from build123d import *

# Parameters (mm, degrees)
CROQUIS1_R              = 2.005138112
SALIENTE_EXTRUIR1_DEPTH = 4
CROQUIS2_W              = 30
CROQUIS2_H              = 5
SALIENTE_EXTRUIR2_DEPTH = 30
CROQUIS3_R              = 1.75
CROQUIS3_R_2            = 4
CORTAR_EXTRUIR1_DEPTH   = 52.778373864
REDONDEO1_R             = 10
REDONDEO2_R             = 5
REDONDEO4_R             = 2
CROQUIS4_R              = 3.4
CORTAR_EXTRUIR2_DEPTH   = 2.25
NERVIO12_REACH          = 56.369
CROQUIS7_WALL_W         = 121.91855764
CROQUIS7_WALL_H         = 5
NERVIO13_REACH          = 56.369
CROQUIS8_WALL_W         = 121.91855764
CROQUIS8_WALL_H         = 5
REDONDEO6_R             = 3
REDONDEO7_R             = 2
REDONDEO8_R             = 1


with BuildPart() as part:
    # Croquis1 → Saliente-Extruir1 (new body)
    with BuildSketch(Plane.XY):
        Polygon((0, 21.15), (0, 30), (30, 30), (30, 21.15), (30, 14.85), (30, 0), (0, 0), (0, 14.85), align=None)
        with Locations((9, 18)):
            Circle(CROQUIS1_R, mode=Mode.SUBTRACT)
        with Locations((21, 18)):
            Circle(CROQUIS1_R, mode=Mode.SUBTRACT)
        with Locations((21, 6)):
            Circle(CROQUIS1_R, mode=Mode.SUBTRACT)
        with Locations((9, 6)):
            Circle(CROQUIS1_R, mode=Mode.SUBTRACT)
    extrude(amount=SALIENTE_EXTRUIR1_DEPTH)

    # Croquis2 → Saliente-Extruir2 (add)
    with BuildSketch(Plane.XY.offset(4)):
        with Locations((15, 27.5)):
            Rectangle(CROQUIS2_W, CROQUIS2_H)
    extrude(amount=SALIENTE_EXTRUIR2_DEPTH)

    # Croquis3 → Cortar-Extruir1 (cut, through all)
    with BuildSketch(Plane.XZ.offset(-25)):
        with Locations(Location((15, 27.25, 0), (0, 0, 270))):
            Circle(CROQUIS3_R)
        with Locations(Location((15, 10.75, 0), (0, 0, 270))):
            Circle(CROQUIS3_R)
        with Locations(Location((15, 19, 0), (0, 0, 270))):
            Circle(CROQUIS3_R_2)
    extrude(amount=-CORTAR_EXTRUIR1_DEPTH, mode=Mode.SUBTRACT)

    # Redondeo1
    redondeo1_edges = [part.edges().sort_by_distance(p)[0] for p in [
        (0, 27.5, 34),
        (30, 27.5, 34),
    ]]
    fillet(redondeo1_edges, radius=REDONDEO1_R)

    # Redondeo2
    redondeo2_edges = [part.edges().sort_by_distance(p)[0] for p in [
        (30, 0, 2),
        (0, 0, 2),
    ]]
    fillet(redondeo2_edges, radius=REDONDEO2_R)

    # Redondeo4
    redondeo4_edges = [part.edges().sort_by_distance(p)[0] for p in [
        (15, 30, 0),
    ]]
    fillet(redondeo4_edges, radius=REDONDEO4_R)

    # Croquis4 → Cortar-Extruir2 (cut)
    with BuildSketch(Plane(origin=(0, 30, 0), x_dir=(1, 0, 0), z_dir=(0, 1, 0))):
        with Locations(Location((15, -10.75, 0), (0, 0, 270))):
            Circle(CROQUIS4_R)
        with Locations(Location((15, -27.25, 0), (0, 0, 270))):
            Circle(CROQUIS4_R)
    extrude(amount=-CORTAR_EXTRUIR2_DEPTH, mode=Mode.SUBTRACT)

    # Croquis7 wall → Nervio12 (add, up to next)
    with BuildSketch(Plane(origin=(30, 20, 6.5), x_dir=(0, -0.894427191, -0.4472135955), z_dir=(0, 0.4472135955, -0.894427191)), mode=Mode.PRIVATE) as nervio12_sk1:
        with Locations((0, 2.5)):
            Rectangle(CROQUIS7_WALL_W, CROQUIS7_WALL_H)
    nervio12_tool1 = extrude(nervio12_sk1.sketch, amount=NERVIO12_REACH, mode=Mode.PRIVATE) - part.part
    add(nervio12_tool1.solids().sort_by_distance((30, 20, 6.5))[0])

    # Croquis8 wall → Nervio13 (add, up to next)
    with BuildSketch(Plane(origin=(0, 20, 6.5), x_dir=(0, 0.894427191, 0.4472135955), z_dir=(0, 0.4472135955, -0.894427191)), mode=Mode.PRIVATE) as nervio13_sk1:
        with Locations((0, 2.5)):
            Rectangle(CROQUIS8_WALL_W, CROQUIS8_WALL_H)
    nervio13_tool1 = extrude(nervio13_sk1.sketch, amount=NERVIO13_REACH, mode=Mode.PRIVATE) - part.part
    add(nervio13_tool1.solids().sort_by_distance((0, 20, 6.5))[0])

    # Redondeo6
    redondeo6_edges = [part.edges().sort_by_distance(p)[0] for p in [
        (27.5, 25, 9),
        (27.5, 15, 4),
        (2.5, 25, 9),
        (2.5, 15, 4),
    ]]
    fillet(redondeo6_edges, radius=REDONDEO6_R)

    # Redondeo7
    redondeo7_edges = [part.edges().sort_by_distance(p)[0] for p in [
        (15, 25, 4),
    ]]
    fillet(redondeo7_edges, radius=REDONDEO7_R)

    # Redondeo8
    redondeo8_edges = [part.edges().sort_by_distance(p)[0] for p in [
        (5, 25, 8.427050983),
        (5, 24.414213562, 4.585786438),
        (5, 18.645898034, 4),
        (25, 25, 8.427050983),
        (25, 24.414213562, 4.585786438),
        (25, 18.645898034, 4),
    ]]
    fillet(redondeo8_edges, radius=REDONDEO8_R)


solid = part.part
Check sheet for the modelled part. Datum: model origin and axes. Units: mm. A direction names the side the tool comes from. Round coordinates to 2 decimals unless told otherwise and drop trailing zeros. Order: outer loops, then holes, each group sorted by start corner. A loop starts at its lowest first (then second) coordinate and runs counter-clockwise, first axis right, second up.
(1) Cross-section at B-B, the plane y = 18. Enter the section's corners in (x, z), and give its area (3 significant figures).
(2) Cross-section at D-D, the plane y = 27.25. Enter the section's corners in (x, z).
(3) Cross-section at A-A, the plane z = 19. Enter the section's corners in (x, y).
(4) Go/stop test with flat-tipped pins: P1, Ø9, axis at x = 15, z = 10.75, coming from the -Y side; P2, Ø1.5, axis at x = 23.5, y = 15, coming from the +Z side; P3, Ø4, axis at x = 15, z = 27.25, coming from the +Y side; P4, Ø2.5, axis at x = 9, y = 18, coming from the +Z side. Record where each tip stops, or that it passes through.
(5) Scan lines: probe 1 along Y at (x, z) = (21, 2.85); probe 2 along X at (y, z) = (27, 10.75); probe 3 along Y at (x, z) = (9, 1). Record each from-to range of solid material in increasing order.
(6) Draft check along X on faces 1 (the flat face through (15, 0, 2)), 2 (the cylindrical face through (5.301, 19.553, 4.285)), 3 (the flat face through (16, 27.75, 9)), 4 (the cylindrical face through (28, 1, 2)). Enter one of: pulls with the +X half, pulls with the -X half, needs draft (parallel to the pull), parting line crosses it, or undercut.
(7) Cross-section at C-C, the plane x = 9. Enter the section's corners in (y, z), and give its area (3 significant figures).
(8) Access from +Z, -Z, +X, -X, +Y, -Y to the whole of each face (thin tool, end or side, straight path). Record for faces 5 (the cylindrical face through (11.68, 28.89, 10.01)), 6 (the flat face through (15, 9, 4)), 7 (the cylindrical face through (7.522, 19.355, 1.972)).
Check sheet entries:
1. outline: (0, 0) - (6.99, 0) - (6.99, 4) - (6, 4) arc R1 cw to (5, 5) - (5, 5.5) - (0, 5.5) - close; (11.01, 0) - (18.99, 0) - (18.99, 4) - (11.01, 4) - close; (23.01, 0) - (30, 0) - (30, 5.5) - (25, 5.5) - (25, 5) arc R1 cw to (24, 4) - (23.01, 4) - close
1. area: 103 mm2
2. outline: (0, 0) - (30, 0) - (30, 24) arc R10 ccw to (20, 34) - (10, 34) arc R10 ccw to (0, 24) - close; hole circle Ø8 at (15, 19); hole circle Ø3.5 at (15, 10.75); hole circle Ø3.5 at (15, 27.25)
3. outline: (0, 25) - (11, 25) - (11, 30) - (0, 30) - close; (19, 25) - (30, 25) - (30, 30) - (19, 30) - close
4. P1: stops at y = 25
4. P2: stops at z = 4.03
4. P3: stops at y = 27.75
4. P4: passes through
5. probe 1: y = 0 to 3.99, 8.01 to 15.99, 20.01 to 30
5. probe 2: x = 0 to 13.25, 16.75 to 30
5. probe 3: y = 0 to 3.99, 8.01 to 15.99, 20.01 to 29.73
6. face 1: needs draft
6. face 2: undercut
6. face 3: undercut
6. face 4: pulls with the +X half
7. outline: (0, 0) - (3.99, 0) - (3.99, 4) - (0, 4) - close; (8.01, 0) - (15.99, 0) - (15.99, 4) - (8.01, 4) - close; (20.01, 0) - (28, 0) arc R2 ccw to (30, 2) - (30, 33.95) - (25, 33.95) - (25, 6) arc R2 cw to (23, 4) - (20.01, 4) - close
7. area: 238 mm2
8. face 5: +Y
8. face 6: +Z, -Y
8. face 7: +Z, -Z
